from build123d import *

# Parameters (mm, degrees)
RECTANGULAR_TUBE_3_X_2_X_0_25_1_DEPTH = 431.8
CUT_EXTRUDE1_DEPTH                    = 221.702469402


with BuildPart() as part:
    # Sketch13 → Rectangular tube 3 X 2 X 0.25(1) (new body)
    with BuildSketch(Plane.ZY.offset(-215.9)):
        with BuildLine():
            Line((-7.9375, -38.1), (7.9375, -38.1))
            ThreePointArc((7.9375, -38.1), (11.305096045, -36.705096045), (12.7, -33.3375))
            Line((12.7, -33.3375), (12.7, 33.3375))
            ThreePointArc((12.7, 33.3375), (11.305096045, 36.705096045), (7.9375, 38.1))
            Line((7.9375, 38.1), (-7.9375, 38.1))
            ThreePointArc((-7.9375, 38.1), (-11.305096045, 36.705096045), (-12.7, 33.3375))
            Line((-12.7, 33.3375), (-12.7, -33.3375))
            ThreePointArc((-12.7, -33.3375), (-11.305096045, -36.705096045), (-7.9375, -38.1))
        make_face()
        with BuildLine():
            Line((-7.9375, -34.925), (7.9375, -34.925))
            ThreePointArc((7.9375, -34.925), (9.060032015, -34.460032015), (9.525, -33.3375))
            Line((9.525, -33.3375), (9.525, 33.3375))
            ThreePointArc((9.525, 33.3375), (9.060032015, 34.460032015), (7.9375, 34.925))
            Line((7.9375, 34.925), (-7.9375, 34.925))
            ThreePointArc((-7.9375, 34.925), (-9.060032015, 34.460032015), (-9.525, 33.3375))
            Line((-9.525, 33.3375), (-9.525, -33.3375))
            ThreePointArc((-9.525, -33.3375), (-9.060032015, -34.460032015), (-7.9375, -34.925))
        make_face(mode=Mode.SUBTRACT)
    extrude(amount=RECTANGULAR_TUBE_3_X_2_X_0_25_1_DEPTH)

    # s → Cut-Extrude1 (cut, through all)
    with BuildSketch(Plane.XY.offset(12.7)):
        Polygon((-215.9, -38.1), (-215.9, 38.1), (-48.694360485, 38.1), align=None)
    extrude(amount=-CUT_EXTRUDE1_DEPTH, mode=Mode.SUBTRACT)


solid = part.part
Geometry: final body of the model. Coordinates: model frame, mm. A direction names the side the tool comes from. Give positions to 0.01 mm unless a question says otherwise; leave off trailing zeros. Write each loop counter-clockwise with the first axis right and the second up, starting at its lowest first coordinate (ties: lowest second). Pieces come first, ordered by that corner, then holes. Notation, with made-up numbers: (56, -4.75) -> (93, -4.75) arc R24 ccw to (93, 6.25) -> close; hole circle Ø7 at (-22, -16). An arc over 180 degrees is marked (long way). Answer in a Markdown table with one row per item.
(1) Section query C-C on x = -20. Return loops of the section in (y, z) (1 decimal).
Answers below:
| item | result |
|---|---|
| outline | (-38.1, -7.9) arc R4.8 ccw to (-33.3, -12.7) -> (33.3, -12.7) arc R4.8 ccw to (38.1, -7.9) -> (38.1, 7.9) arc R4.8 ccw to (33.3, 12.7) -> (-33.3, 12.7) arc R4.8 ccw to (-38.1, 7.9) -> close; hole (-34.9, -7.9) arc R1.6 ccw to (-33.3, -9.5) -> (33.3, -9.5) arc R1.6 ccw to (34.9, -7.9) -> (34.9, 7.9) arc R1.6 ccw to (33.3, 9.5) -> (-33.3, 9.5) arc R1.6 ccw to (-34.9, 7.9) -> close |
(2) Ray query, line 1 along Z through (x, y) = (-116.5, -6) (3 decimals); line 2 along Y through (x, z) = (29, -5) (3 decimals); line 3 along Y through (x, z) = (-96.5, -0.25) (3 decimals). Return the intervals inside material, ascending. Write a range as [from, to].
Answers below:
| item | result |
|---|---|
| line 1 | [-12.7, -9.525], [9.525, 12.7] |
| line 2 | [-38.1, -34.925], [34.925, 38.1] |
| line 3 | [-38.1, -34.925] |
(3) Section query B-B on z = -0.25. Return loops of the section in (x, y) (3 decimals).
Answers below:
| item | result |
|---|---|
| outline | (-215.9, -38.1) -> (215.9, -38.1) -> (215.9, -34.925) -> (-208.933, -34.925) -> close; (-55.661, 34.925) -> (215.9, 34.925) -> (215.9, 38.1) -> (-48.694, 38.1) -> close |
(4) Pin query (flat end, axial travel): pin 1 (8 mm diameter, centred on x = -51.5, z = -1.5, fed in from +Y); pin 2 (3 mm diameter, centred on x = 56, z = -10, fed in from -Y); pin 3 (8 mm diameter, centred on x = -162.5, z = -0.5, fed in from +Y) (3 decimals). Return the tip coordinate at first contact, or that it passes through.
Answers below:
| item | result |
|---|---|
| pin 1 | y = 38.1 |
| pin 2 | y = -38.07 |
| pin 3 | y = -34.925 |
(5) Set-up query: faces 1 (the flat face through (215.9, 0, -10)), 2 (the flat face through (82, 34.925, 0)). Return all of +Z, -Z, +X, -X, +Y, -Y with unobstructed straight access to the full face (end or side cutting, diameter ignored); none if empty.
Answers below:
| item | result |
|---|---|
| face 1 | +Z, -Z, +X, +Y, -Y |
| face 2 | +X, -X |
(6) Section query D-D on x = -170.5. Return loops of the section in (y, z) (1 decimal).
Answers below:
| item | result |
|---|---|
| outline | (-38.1, -7.9) arc R4.8 ccw to (-33.3, -12.7) -> (-17.4, -12.7) -> (-17.4, -9.5) -> (-33.3, -9.5) arc R1.6 cw to (-34.9, -7.9) -> (-34.9, 7.9) arc R1.6 cw to (-33.3, 9.5) -> (-17.4, 9.5) -> (-17.4, 12.7) -> (-33.3, 12.7) arc R4.8 ccw to (-38.1, 7.9) -> close |
(7) Section query A-A on y = -18.5. Return loops of the section in (x, z) (3 decimals), then the cut area to 3 significant figures.
Answers below:
| item | result |
|---|---|
| outline | (-172.892, -12.7) -> (215.9, -12.7) -> (215.9, -9.525) -> (-172.892, -9.525) -> close; (-172.892, 9.525) -> (215.9, 9.525) -> (215.9, 12.7) -> (-172.892, 12.7) -> close |
| area | 2,470 mm^2 |
(8) Draft query along Y for faces 3 (the flat face through (55, 0, 12.7)), 4 (the flat face through (3, -38.1, 0)), 5 (the flat face through (6, -34.925, 0)). Return one class per face: +Y half, -Y half, draft (parallel to the pull), parting line (faces both ways), or undercut.
Answers below:
| item | result |
|---|---|
| face 3 | draft |
| face 4 | -Y half |
| face 5 | undercut |
